Verification items for the finished model (mm, model axes). A direction names the side the tool comes from. Round coordinates to 2 decimals unless told otherwise and drop trailing zeros. Loops run counter-clockwise (first coordinate to the right, second up) from the corner with the lowest first, then second, coordinate; pieces in that order, holes last. Notation, with made-up numbers: M 69.5,-26 L 80.5,-26 A20 cw 80.5,2 Z; hole C 35,28.25 d1. An arc over 180 degrees is marked long. Answer as CSV lines item,"result".
Autodesk Inventor part; units mm, degrees
ref_plane "YZ Plane" through (0, 0, 0) normal (1, 0, 0) x (0, 1, 0)
ref_plane "XZ Plane" through (0, 0, 0) normal (0, 1, 0) x (-1, 0, 0)
ref_plane "XY Plane" through (0, 0, 0) normal (0, 0, 1) x (1, 0, 0)
sketch "Esboço1" plane through (0, 0, 0) normal (0, 0, 1) x (1, 0, 0)
  circle A0 centre (0, 0) radius 12.5
  circle A1 centre (0, 0) radius 15
  dimension "d0" = 25
  dimension "d1" = 30
extrude "Extrusão1" add sketch "Esboço1" along normal blind 11
sketch "Esboço2" plane through (0, 0, 11) normal (0, 0, 1) x (1, 0, 0)
  circle A0 centre (0, 0) radius 15
  dimension "d4" = 30
extrude "Extrusão2" add sketch "Esboço2" against normal blind 3
sketch "Esboço4" plane through (0, 0, 11) normal (0, 0, 1) x (1, 0, 0)
  circle A0 centre (0, 0) radius 11
  dimension "d10" = 22
extrude "Extrusão4" add sketch "Esboço4" along normal blind 16
sketch "Esboço5" plane through (0, 0, 27) normal (0, 0, 1) x (1, 0, 0)
  circle A0 centre (0, 0) radius 7.5
  dimension "d13" = 15
extrude "Extrusão5" cut sketch "Esboço5" against normal through all
sketch "Esboço6" plane through (0, 0, 27) normal (0, 0, 1) x (1, 0, 0)
  circle A0 centre (0, 0) radius 10
  circle A1 centre (0, 0) radius 8
  circle A2 centre (0, 0) radius 7.5
  circle A3 centre (0, 0) radius 11
  dimension "d16" = 20
  dimension "d27" = 16
  dimension "d28" = 22
extrude "Extrusão6" cut sketch "Esboço6" against normal blind 5
thread "Rosca1"
sketch "Esboço7" plane through (0, 0, 0) normal (0, 1, 0) x (-1, 0, 0)
  line L0 (4.5, 22) -> (-4.5, 22)
  line L1 (-4.5, 22) -> (-4.5, 27)
  line L2 (-4.5, 27) -> (4.5, 27)
  line L3 (4.5, 27) -> (4.5, 22)
  line L4 (4.5, 22) -> (-4.5, 27) construction
  line L5 (-4.5, 22) -> (4.5, 27) construction
  line L6 (10, 27) -> (-10, 27)
  point P0 (0, 0)
  point P1 (0, 24.5)
  dimension "d22" = 9
  dimension "d23" = 5
  dimension "d24" = 0
extrude "Extrusão7" cut sketch "Esboço7" along normal through all both and the other way through all
sketch "Esboço8" plane through (0, 0, 22) normal (0, 0, 1) x (1, 0, 0)
  line L0 (-10.5, 10.5) -> (10.5, 10.5)
  line L1 (10.5, 10.5) -> (10.5, -10.5)
  line L2 (10.5, -10.5) -> (-10.5, -10.5)
  line L3 (-10.5, -10.5) -> (-10.5, 10.5)
  line L4 (-10.5, 10.5) -> (10.5, -10.5) construction
  line L5 (10.5, 10.5) -> (-10.5, -10.5) construction
  circle A0 centre (0, 0) radius 11
  point P0 (-3.2787, -10.5)
  point P1 (3.2787, -10.5)
  point P2 (3.2787, 10.5)
  point P3 (-3.2787, 10.5)
  dimension "d29" = 21
  dimension "d30" = 21
  dimension "d31" = 22
extrude "Extrusão8" cut sketch "Esboço8" against normal blind 11 contours A0 L0 | L2 A0
properties part number "CARCAÇA DO BOTÃO"
1) Set-up check for faces 1 (the cylindrical face through (-8, 0, 25)), 2 (the cylindrical face through (11, 0, 16)), 3 (the flat face through (4.5, 8, 24)), 4 (the flat face through (0, 10.5, 17)): record each of +Z, -Z, +X, -X, +Y, -Y from which the full face is reachable in a straight line by a thin tool's end or side.
Here are the results:
face 1,"+Z"
face 2,"+Z, +X"
face 3,"+Z, +Y, -Y"
face 4,"+Z, +X, -X, +Y"
2) Section check C-C (y = 0). Record the cut outline in (x, z), plus the area to 3 significant figures.
Here are the results:
outline,"M -15,0 L -12.5,0 L -12.5,8 L -7.5,8 L -7.5,22 L -8,22 L -8,27 L -10,27 L -10,22 L -11,22 L -11,11 L -15,11 Z; M 7.5,8 L 12.5,8 L 12.5,0 L 15,0 L 15,11 L 11,11 L 11,22 L 10,22 L 10,27 L 8,27 L 8,22 L 7.5,22 Z"
area,"182 mm^2"
3) Section check A-A (z = 23). Record the cut outline in (x, y).
Here are the results:
outline,"M -4.5,-8.93 L -4.5,-6.61 A8 cw -4.5,6.61 L -4.5,8.93 A10 ccw Z; M 4.5,-8.93 A10 ccw 4.5,8.93 L 4.5,6.61 A8 cw 4.5,-6.61 Z"
4) Go/stop test with flat-tipped pins: pin 1 (12.5 mm diameter, centred on x = -5.5, y = 5, fed in from -Z); pin 2 (10 mm diameter, centred on x = -7.5, z = 22, fed in from +Y); pin 3 (0.7 mm diameter, centred on y = 7.5, z = 25, fed in from -X); pin 4 (1.5 mm diameter, centred on y = -6.5, z = 7.5, fed in from +X). Record where each tip stops, or that it passes through.
Here are the results:
pin 1,"stops at z = 0"
pin 2,"stops at y = 10.5"
pin 3,"stops at x = -6.99"
pin 4,"stops at x = 13.85"
5) Section check D-D (z = 19.75). Record the cut outline in (x, y).
Here are the results:
outline,"M -3.28,-10.5 L 3.28,-10.5 A11 ccw 3.28,10.5 L -3.28,10.5 A11 ccw Z; hole C 0,0 d15"
6) Section check B-B (x = 0). Record the cut outline in (y, z).
Here are the results:
outline,"M -15,0 L -12.5,0 L -12.5,8 L -7.5,8 L -7.5,22 L -10.5,22 L -10.5,11 L -15,11 Z; M 7.5,8 L 12.5,8 L 12.5,0 L 15,0 L 15,11 L 10.5,11 L 10.5,22 L 7.5,22 Z"
7) Material ranges on probe 1 along X at (y, z) = (0, 13.75); probe 2 along Y at (x, z) = (0, 4); probe 3 along Y at (x, z) = (0, 15), recorded low to high.
Here are the results:
probe 1,"x = -11 to -7.5, 7.5 to 11"
probe 2,"y = -15 to -12.5, 12.5 to 15"
probe 3,"y = -10.5 to -7.5, 7.5 to 10.5"
